Design review of the part built by this model. Coordinates are the model's own, in mm. Face numbers are marked on the shaded views. Coordinates: 2 decimals unless noted, no trailing zeros. Order: outer loops, then holes, each group sorted by start corner. A loop starts at its lowest first (then second) coordinate and runs counter-clockwise, first axis right, second up. Notation, with made-up numbers: M 41,80 L 91,80 A24 cw 91,96 Z; hole C 4,18 d9. An arc over 180 degrees is marked long. Answer in a Markdown table with one row per item.
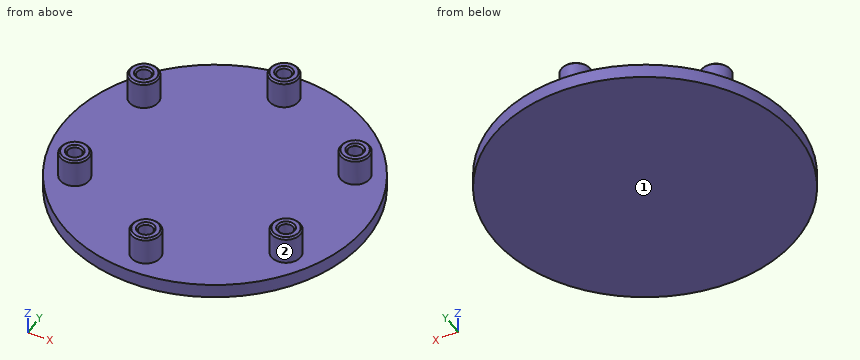
from build123d import *
from OCP.BRepFilletAPI import BRepFilletAPI_MakeChamfer

# Parameters (mm, degrees)
SKETCH1_R                     = 34.29
BOSS_EXTRUDE1_DEPTH           = 3.175
SKETCH2_R                     = 3.302
BOSS_EXTRUDE2_DEPTH           = 6.35
SKETCH3_R                     = 1.5875
CUT_EXTRUDE1_DEPTH            = 4.572
CUT_EXTRUDE1_DRAFT            = -1
CHAMFER1_SIZE                 = 0.381
CHAMFER1_SIZE2                = 0.387827593
CIRPATTERN1_COUNT             = 6
CIRPATTERN1_COPY_1_SKETCH_R   = 1.5875
CIRPATTERN1_COPY_1_DEPTH      = 4.572
CIRPATTERN1_COPY_1_DRAFT      = -1
CIRPATTERN1_COPY_2_SKETCH_R   = 1.5875
CIRPATTERN1_COPY_2_DEPTH      = 4.572
CIRPATTERN1_COPY_2_DRAFT      = -1
CIRPATTERN1_COPY_3_SKETCH_R   = 1.5875
CIRPATTERN1_COPY_3_DEPTH      = 4.572
CIRPATTERN1_COPY_3_DRAFT      = -1
CIRPATTERN1_COPY_4_SKETCH_R   = 1.5875
CIRPATTERN1_COPY_4_DEPTH      = 4.572
CIRPATTERN1_COPY_4_DRAFT      = -1
CIRPATTERN1_COPY_5_SKETCH_R   = 1.5875
CIRPATTERN1_COPY_5_DEPTH      = 4.572
CIRPATTERN1_COPY_5_DRAFT      = -1
CHAMFER1_OF_CIRPATTERN1_SIZE  = 0.381
CHAMFER1_OF_CIRPATTERN1_SIZE2 = 0.387827593


with BuildPart() as part:
    # Sketch1 → Boss-Extrude1 (new body)
    with BuildSketch(Plane.XY):
        Circle(SKETCH1_R)
    extrude(amount=BOSS_EXTRUDE1_DEPTH)

    # Sketch2 → Boss-Extrude2 (add)
    with BuildSketch(Plane.XY.offset(3.175)):
        with Locations((0, 27.94)):
            Circle(SKETCH2_R)
    boss_extrude2 = extrude(amount=BOSS_EXTRUDE2_DEPTH)


with BuildPart() as cut_extrude1_tool:
    # Sketch3 → Cut-Extrude1 (with draft: the straight prism first)
    with BuildSketch(Plane.XY.offset(9.525)):
        with Locations((0, 27.94)):
            Circle(SKETCH3_R)
    extrude(amount=-CUT_EXTRUDE1_DEPTH)
    # Cut-Extrude1: the draft: its side faces are tilted about the plane it starts from
    cut_extrude1_sides = [cut_extrude1_tool.faces().sort_by_distance(p)[0] for p in [
        (-1.5875, 27.94, 7.239),
    ]]
    draft(cut_extrude1_sides, Plane.XY.offset(9.525), CUT_EXTRUDE1_DRAFT)


with BuildPart() as part_1:
    add(part.part)

    # Cut-Extrude1: cut by cut_extrude1_tool
    add(cut_extrude1_tool.part, mode=Mode.SUBTRACT)

    # Chamfer1: one chamfer whose edges measure the first distance from different faces: ONE call of the kernel's chamfer builder (chamfer() names one face for all edges)
    chamfer1_edges_1 = [part_1.edges().sort_by_distance(p)[0] for p in [
        (-1.5875, 27.94, 9.525),
    ]]
    chamfer1_side_1 = [part_1.faces().sort_by_distance(p)[0] for p in [
        (-3.208605336, 27.94, 9.525),
    ]]
    chamfer1_edges_2 = [part_1.edges().sort_by_distance(p)[0] for p in [
        (-3.302, 27.94, 9.525),
    ]]
    chamfer1 = BRepFilletAPI_MakeChamfer(part_1.part.solid().wrapped)
    for e in chamfer1_edges_1:
        chamfer1.Add(CHAMFER1_SIZE, CHAMFER1_SIZE2, e.wrapped, chamfer1_side_1[0].wrapped)  # the first distance lies on this face
    for e in chamfer1_edges_2:
        chamfer1.Add(CHAMFER1_SIZE, e.wrapped)
    add(Compound.cast(chamfer1.Shape()), mode=Mode.REPLACE)

    # CirPattern1: Boss-Extrude2 ×6 about axis
    cirpattern1_axis = Axis((0, 0, 0), (0, 0, 1))
    for i in range(1, CIRPATTERN1_COUNT):
        add(boss_extrude2.rotate(cirpattern1_axis, i * 360 / CIRPATTERN1_COUNT))


with BuildPart() as cirpattern1_copy_1_tool:
    # CirPattern1 copy 1 sketch → CirPattern1 copy 1 (with draft: the straight prism first)
    with BuildSketch(Plane(origin=(0, 0, 9.525), x_dir=(0.5000000000000001, 0.8660254037844386, 0), z_dir=(0, 0, 1))):
        with Locations((0, 27.94)):
            Circle(CIRPATTERN1_COPY_1_SKETCH_R)
    extrude(amount=-CIRPATTERN1_COPY_1_DEPTH)
    # CirPattern1 copy 1: the draft: its side faces are tilted about the plane it starts from
    cirpattern1_copy_1_sides = [cirpattern1_copy_1_tool.faces().sort_by_distance(p)[0] for p in [
        (-24.990499782, 12.595184671, 7.239),
    ]]
    draft(cirpattern1_copy_1_sides, Plane(origin=(0, 0, 9.525), x_dir=(0.5000000000000001, 0.8660254037844386, 0), z_dir=(0, 0, 1)), CIRPATTERN1_COPY_1_DRAFT)


with BuildPart() as part_2:
    add(part_1.part)

    # CirPattern1 copy 1: cut by cirpattern1_copy_1_tool
    add(cirpattern1_copy_1_tool.part, mode=Mode.SUBTRACT)


with BuildPart() as cirpattern1_copy_2_tool:
    # CirPattern1 copy 2 sketch → CirPattern1 copy 2 (with draft: the straight prism first)
    with BuildSketch(Plane(origin=(0, 0, 9.525), x_dir=(-0.4999999999999998, 0.8660254037844387, 0), z_dir=(0, 0, 1))):
        with Locations((0, 27.94)):
            Circle(CIRPATTERN1_COPY_2_SKETCH_R)
    extrude(amount=-CIRPATTERN1_COPY_2_DEPTH)
    # CirPattern1 copy 2: the draft: its side faces are tilted about the plane it starts from
    cirpattern1_copy_2_sides = [cirpattern1_copy_2_tool.faces().sort_by_distance(p)[0] for p in [
        (-23.402999782, -15.344815329, 7.239),
    ]]
    draft(cirpattern1_copy_2_sides, Plane(origin=(0, 0, 9.525), x_dir=(-0.4999999999999998, 0.8660254037844387, 0), z_dir=(0, 0, 1)), CIRPATTERN1_COPY_2_DRAFT)


with BuildPart() as part_3:
    add(part_2.part)

    # CirPattern1 copy 2: cut by cirpattern1_copy_2_tool
    add(cirpattern1_copy_2_tool.part, mode=Mode.SUBTRACT)


with BuildPart() as cirpattern1_copy_3_tool:
    # CirPattern1 copy 3 sketch → CirPattern1 copy 3 (with draft: the straight prism first)
    with BuildSketch(Plane(origin=(0, 0, 9.525), x_dir=(-1, 0, 0), z_dir=(0, 0, 1))):
        with Locations((0, 27.94)):
            Circle(CIRPATTERN1_COPY_3_SKETCH_R)
    extrude(amount=-CIRPATTERN1_COPY_3_DEPTH)
    # CirPattern1 copy 3: the draft: its side faces are tilted about the plane it starts from
    cirpattern1_copy_3_sides = [cirpattern1_copy_3_tool.faces().sort_by_distance(p)[0] for p in [
        (1.5875, -27.94, 7.239),
    ]]
    draft(cirpattern1_copy_3_sides, Plane(origin=(0, 0, 9.525), x_dir=(-1, 0, 0), z_dir=(0, 0, 1)), CIRPATTERN1_COPY_3_DRAFT)


with BuildPart() as part_4:
    add(part_3.part)

    # CirPattern1 copy 3: cut by cirpattern1_copy_3_tool
    add(cirpattern1_copy_3_tool.part, mode=Mode.SUBTRACT)


with BuildPart() as cirpattern1_copy_4_tool:
    # CirPattern1 copy 4 sketch → CirPattern1 copy 4 (with draft: the straight prism first)
    with BuildSketch(Plane(origin=(0, 0, 9.525), x_dir=(-0.5000000000000004, -0.8660254037844384, 0), z_dir=(0, 0, 1))):
        with Locations((0, 27.94)):
            Circle(CIRPATTERN1_COPY_4_SKETCH_R)
    extrude(amount=-CIRPATTERN1_COPY_4_DEPTH)
    # CirPattern1 copy 4: the draft: its side faces are tilted about the plane it starts from
    cirpattern1_copy_4_sides = [cirpattern1_copy_4_tool.faces().sort_by_distance(p)[0] for p in [
        (24.990499782, -12.595184671, 7.239),
    ]]
    draft(cirpattern1_copy_4_sides, Plane(origin=(0, 0, 9.525), x_dir=(-0.5000000000000004, -0.8660254037844384, 0), z_dir=(0, 0, 1)), CIRPATTERN1_COPY_4_DRAFT)


with BuildPart() as part_5:
    add(part_4.part)

    # CirPattern1 copy 4: cut by cirpattern1_copy_4_tool
    add(cirpattern1_copy_4_tool.part, mode=Mode.SUBTRACT)


with BuildPart() as cirpattern1_copy_5_tool:
    # CirPattern1 copy 5 sketch → CirPattern1 copy 5 (with draft: the straight prism first)
    with BuildSketch(Plane(origin=(0, 0, 9.525), x_dir=(0.5000000000000001, -0.8660254037844386, 0), z_dir=(0, 0, 1))):
        with Locations((0, 27.94)):
            Circle(CIRPATTERN1_COPY_5_SKETCH_R)
    extrude(amount=-CIRPATTERN1_COPY_5_DEPTH)
    # CirPattern1 copy 5: the draft: its side faces are tilted about the plane it starts from
    cirpattern1_copy_5_sides = [cirpattern1_copy_5_tool.faces().sort_by_distance(p)[0] for p in [
        (23.402999782, 15.344815329, 7.239),
    ]]
    draft(cirpattern1_copy_5_sides, Plane(origin=(0, 0, 9.525), x_dir=(0.5000000000000001, -0.8660254037844386, 0), z_dir=(0, 0, 1)), CIRPATTERN1_COPY_5_DRAFT)


with BuildPart() as part_6:
    add(part_5.part)

    # CirPattern1 copy 5: cut by cirpattern1_copy_5_tool
    add(cirpattern1_copy_5_tool.part, mode=Mode.SUBTRACT)

    # Chamfer1 of CirPattern1: one chamfer whose edges measure the first distance from different faces: ONE call of the kernel's chamfer builder (chamfer() names one face for all edges)
    chamfer1_of_cirpattern1_edges_1 = [part_6.edges().sort_by_distance(p)[0] for p in [
        (-24.990499782, 12.595184671, 9.525),
    ]]
    chamfer1_of_cirpattern1_side_1 = [part_6.faces().sort_by_distance(p)[0] for p in [
        (-25.80105245, 11.191266268, 9.525),
    ]]
    chamfer1_of_cirpattern1_edges_2 = [part_6.edges().sort_by_distance(p)[0] for p in [
        (-25.847749782, 11.110384117, 9.525),
    ]]
    chamfer1_of_cirpattern1_edges_3 = [part_6.edges().sort_by_distance(p)[0] for p in [
        (-23.402999782, -15.344815329, 9.525),
    ]]
    chamfer1_of_cirpattern1_side_3 = [part_6.faces().sort_by_distance(p)[0] for p in [
        (-22.592447114, -16.748733732, 9.525),
    ]]
    chamfer1_of_cirpattern1_edges_4 = [part_6.edges().sort_by_distance(p)[0] for p in [
        (-22.545749782, -16.829615883, 9.525),
    ]]
    chamfer1_of_cirpattern1_edges_5 = [part_6.edges().sort_by_distance(p)[0] for p in [
        (1.5875, -27.94, 9.525),
    ]]
    chamfer1_of_cirpattern1_side_5 = [part_6.faces().sort_by_distance(p)[0] for p in [
        (3.208605336, -27.94, 9.525),
    ]]
    chamfer1_of_cirpattern1_edges_6 = [part_6.edges().sort_by_distance(p)[0] for p in [
        (3.302, -27.94, 9.525),
    ]]
    chamfer1_of_cirpattern1_edges_7 = [part_6.edges().sort_by_distance(p)[0] for p in [
        (24.990499782, -12.595184671, 9.525),
    ]]
    chamfer1_of_cirpattern1_side_7 = [part_6.faces().sort_by_distance(p)[0] for p in [
        (25.80105245, -11.191266268, 9.525),
    ]]
    chamfer1_of_cirpattern1_edges_8 = [part_6.edges().sort_by_distance(p)[0] for p in [
        (25.847749782, -11.110384117, 9.525),
    ]]
    chamfer1_of_cirpattern1_edges_9 = [part_6.edges().sort_by_distance(p)[0] for p in [
        (23.402999782, 15.344815329, 9.525),
    ]]
    chamfer1_of_cirpattern1_side_9 = [part_6.faces().sort_by_distance(p)[0] for p in [
        (22.592447114, 16.748733732, 9.525),
    ]]
    chamfer1_of_cirpattern1_edges_10 = [part_6.edges().sort_by_distance(p)[0] for p in [
        (22.545749782, 16.829615883, 9.525),
    ]]
    chamfer1_of_cirpattern1 = BRepFilletAPI_MakeChamfer(part_6.part.solid().wrapped)
    for e in chamfer1_of_cirpattern1_edges_1:
        chamfer1_of_cirpattern1.Add(CHAMFER1_OF_CIRPATTERN1_SIZE, CHAMFER1_OF_CIRPATTERN1_SIZE2, e.wrapped, chamfer1_of_cirpattern1_side_1[0].wrapped)  # the first distance lies on this face
    for e in chamfer1_of_cirpattern1_edges_2:
        chamfer1_of_cirpattern1.Add(CHAMFER1_OF_CIRPATTERN1_SIZE, e.wrapped)
    for e in chamfer1_of_cirpattern1_edges_3:
        chamfer1_of_cirpattern1.Add(CHAMFER1_OF_CIRPATTERN1_SIZE, CHAMFER1_OF_CIRPATTERN1_SIZE2, e.wrapped, chamfer1_of_cirpattern1_side_3[0].wrapped)  # the first distance lies on this face
    for e in chamfer1_of_cirpattern1_edges_4:
        chamfer1_of_cirpattern1.Add(CHAMFER1_OF_CIRPATTERN1_SIZE, e.wrapped)
    for e in chamfer1_of_cirpattern1_edges_5:
        chamfer1_of_cirpattern1.Add(CHAMFER1_OF_CIRPATTERN1_SIZE, CHAMFER1_OF_CIRPATTERN1_SIZE2, e.wrapped, chamfer1_of_cirpattern1_side_5[0].wrapped)  # the first distance lies on this face
    for e in chamfer1_of_cirpattern1_edges_6:
        chamfer1_of_cirpattern1.Add(CHAMFER1_OF_CIRPATTERN1_SIZE, e.wrapped)
    for e in chamfer1_of_cirpattern1_edges_7:
        chamfer1_of_cirpattern1.Add(CHAMFER1_OF_CIRPATTERN1_SIZE, CHAMFER1_OF_CIRPATTERN1_SIZE2, e.wrapped, chamfer1_of_cirpattern1_side_7[0].wrapped)  # the first distance lies on this face
    for e in chamfer1_of_cirpattern1_edges_8:
        chamfer1_of_cirpattern1.Add(CHAMFER1_OF_CIRPATTERN1_SIZE, e.wrapped)
    for e in chamfer1_of_cirpattern1_edges_9:
        chamfer1_of_cirpattern1.Add(CHAMFER1_OF_CIRPATTERN1_SIZE, CHAMFER1_OF_CIRPATTERN1_SIZE2, e.wrapped, chamfer1_of_cirpattern1_side_9[0].wrapped)  # the first distance lies on this face
    for e in chamfer1_of_cirpattern1_edges_10:
        chamfer1_of_cirpattern1.Add(CHAMFER1_OF_CIRPATTERN1_SIZE, e.wrapped)
    add(Compound.cast(chamfer1_of_cirpattern1.Shape()), mode=Mode.REPLACE)


solid = part_6.part
(1) Draft analysis for pull direction Y (two halves, no side actions). For the marked faces 1 and 2, state which applies: pulls with the +Y half, pulls with the -Y half, needs draft (parallel to the pull), parting line crosses it, or undercut.
Return value:
| item | result |
|---|---|
| face 1 | needs draft |
| face 2 | undercut |
(2) Add section D-D, the plane x = 9. Give the boundary of the cut face in (y, z) (3 decimals), and give its area (3 significant figures).
Return value:
| item | result |
|---|---|
| outline | M -33.088,0 L 33.088,0 L 33.088,3.175 L -33.088,3.175 Z |
| area | 210 mm2 |
(3) For line 1 along Z through (x, y) = (-20.5, 14) (3 decimals); line 2 along Y through (x, z) = (-1, 6.75); line 3 along Y through (x, z) = (23, 8), list the stretches that pass through material, from the lowest coordinate up. Write a range as from..to.
Return value:
| item | result |
|---|---|
| line 1 | z = 0..3.175 |
| line 2 | y = -31.09..-29.11, -26.77..-24.79, 24.79..26.77, 29.11..31.09 |
| line 3 | y = -17.05..-14.97, -12.97..-10.89, 10.89..12.97, 14.97..17.05 |
(4) Add section A-A, the plane z = 6.25. Give the number of separate pieces and of enclosed holes in the cut face, and give its area (3 significant figures).
Return value:
| item | result |
|---|---|
| separate pieces | 6 |
| enclosed holes | 6 |
| area | 161 mm2 |
(5) Add section B-B, the plane y = -19.5. Give the boundary of the cut face in (x, z) (3 decimals).
Return value:
| item | result |
|---|---|
| outline | M -28.206,0 L 28.206,0 L 28.206,3.175 L -28.206,3.175 Z |
(6) Add section C-C, the plane z = 1.5. Give the boundary of the cut face in (x, y).
Return value:
| item | result |
|---|---|
| outline | C 0,0 d68.58 |
(7) Insertion check: pin 1 Ø20.5 at (x, y) = (7.5, -3.5) entering from +Z (3 decimals); pin 2 Ø2.5 at (x, y) = (0, -28.5) entering from +Z; pin 3 Ø5 at (y, z) = (6, 1) entering from +X; pin 4 Ø4 at (y, z) = (-7, 7.5) entering from -X. Each pin has a flat end and moves straight along its axis. Give the tip position at first contact, or say it passes through.
Return value:
| item | result |
|---|---|
| pin 1 | stops at z = 3.175 |
| pin 2 | stops at z = 9.37 |
| pin 3 | stops at x = 34.11 |
| pin 4 | passes through |
